Source: CAD feature listing. Evaluate the final solid. Frame: model axes, mm. A direction names the side the tool comes from. Give positions to 0.01 mm unless a question says otherwise; leave off trailing zeros. Write each loop counter-clockwise with the first axis right and the second up, starting at its lowest first coordinate (ties: lowest second). Pieces come first, ordered by that corner, then holes.
```python
from build123d import *

# Parameters (mm, degrees)
ESQUISSE1_W              = 35.4
ESQUISSE1_H              = 35.4
BOSS_EXTRU_1_DEPTH       = 14
ESQUISSE2_W              = 27.4
ESQUISSE2_H              = 27.4
ENL_V_MAT_EXTRU_1_DEPTH  = 12
ESQUISSE4_R              = 3.25
ESQUISSE4_R_2            = 1.9
BOSS_EXTRU_2_DEPTH       = 4.8
ESQUISSE5_R              = 1.75
ENL_V_MAT_EXTRU_2_DEPTH  = 2
CONG_6_R                 = 2
ESQUISSE9_W              = 1.5
ESQUISSE9_H              = 5.2
ENL_V_MAT_EXTRU_9_DEPTH  = 4
ESQUISSE8_W              = 1.5
ESQUISSE8_H              = 5.2
ENL_V_MAT_EXTRU_10_DEPTH = 4
ESQUISSE7_W              = 1.5
ESQUISSE7_H              = 5.2
ENL_V_MAT_EXTRU_11_DEPTH = 4
ESQUISSE6_W              = 1.5
ESQUISSE6_H              = 5.2
ENL_V_MAT_EXTRU_12_DEPTH = 4
ESQUISSE10_W             = 8.819289119
ESQUISSE10_H             = 5.2
ENL_V_MAT_EXTRU_13_DEPTH = 6


with BuildPart() as part:
    # Esquisse1 → Boss.-Extru.1 (new body)
    with BuildSketch(Plane(origin=(0, 0, 0), x_dir=(1, 0, 0), z_dir=(0, 1, 0))):
        Rectangle(ESQUISSE1_W, ESQUISSE1_H)
    extrude(amount=BOSS_EXTRU_1_DEPTH)

    # Esquisse2 → Enlèv. mat.-Extru.1 (cut)
    with BuildSketch(Plane(origin=(0, 14, 0), x_dir=(1, 0, 0), z_dir=(0, 1, 0))):
        Rectangle(ESQUISSE2_W, ESQUISSE2_H)
    extrude(amount=-ENL_V_MAT_EXTRU_1_DEPTH, mode=Mode.SUBTRACT)

    # Esquisse4 → Boss.-Extru.2 (add)
    # profile 1 of 4: a face of its own
    with BuildSketch(Plane(origin=(0, 2, 0), x_dir=(1, 0, 0), z_dir=(0, 1, 0))):
        with Locations(Location((-10.16, 10.16, 0), (0, 0, 270))):
            Circle(ESQUISSE4_R)
        with Locations(Location((-10.16, 10.16, 0), (0, 0, 270))):
            Circle(ESQUISSE4_R_2, mode=Mode.SUBTRACT)
    # profile 2 of 4: a face of its own
    with BuildSketch(Plane(origin=(0, 2, 0), x_dir=(1, 0, 0), z_dir=(0, 1, 0))):
        with Locations(Location((10.16, 10.16, 0), (0, 0, 270))):
            Circle(ESQUISSE4_R)
        with Locations(Location((10.16, 10.16, 0), (0, 0, 270))):
            Circle(ESQUISSE4_R_2, mode=Mode.SUBTRACT)
    # profile 3 of 4: a face of its own
    with BuildSketch(Plane(origin=(0, 2, 0), x_dir=(1, 0, 0), z_dir=(0, 1, 0))):
        with Locations(Location((10.16, -10.16, 0), (0, 0, 270))):
            Circle(ESQUISSE4_R)
        with Locations(Location((10.16, -10.16, 0), (0, 0, 270))):
            Circle(ESQUISSE4_R_2, mode=Mode.SUBTRACT)
    # profile 4 of 4: a face of its own
    with BuildSketch(Plane(origin=(0, 2, 0), x_dir=(1, 0, 0), z_dir=(0, 1, 0))):
        with Locations(Location((-10.16, -10.16, 0), (0, 0, 270))):
            Circle(ESQUISSE4_R)
        with Locations(Location((-10.16, -10.16, 0), (0, 0, 270))):
            Circle(ESQUISSE4_R_2, mode=Mode.SUBTRACT)
    extrude(amount=BOSS_EXTRU_2_DEPTH)

    # Esquisse5 → Enlèv. mat.-Extru.2 (cut)
    with BuildSketch(Plane(origin=(0, 14, 0), x_dir=(1, 0, 0), z_dir=(0, 1, 0))):
        with Locations(Location((15.5, 15.5, 0), (0, 0, 270))):
            Circle(ESQUISSE5_R)
        with Locations(Location((-15.5, 15.5, 0), (0, 0, 270))):
            Circle(ESQUISSE5_R)
        with Locations(Location((-15.5, -15.5, 0), (0, 0, 270))):
            Circle(ESQUISSE5_R)
        with Locations(Location((15.5, -15.5, 0), (0, 0, 270))):
            Circle(ESQUISSE5_R)
    extrude(amount=-ENL_V_MAT_EXTRU_2_DEPTH, mode=Mode.SUBTRACT)

    # Congé6
    cong_6_edges = [part.edges().sort_by_distance(p)[0] for p in [
        (0, 0, 17.7),
        (-17.7, 0, 0),
        (0, 0, -17.7),
        (17.7, 0, 0),
        (17.7, 7, 17.7),
        (-17.7, 7, 17.7),
        (-17.7, 7, -17.7),
        (17.7, 7, -17.7),
    ]]
    fillet(cong_6_edges, radius=CONG_6_R)

    # Esquisse9 → Enlèv. mat.-Extru.9 (cut)
    with BuildSketch(Plane(origin=(0, 0, -17.7), x_dir=(-1, 0, 0), z_dir=(0, 0, -1))):
        with Locations((-10.95, 9.4)):
            Rectangle(ESQUISSE9_W, ESQUISSE9_H)
        with Locations((-7.3, 9.4)):
            Rectangle(ESQUISSE9_W, ESQUISSE9_H)
        with Locations((-3.65, 9.4)):
            Rectangle(ESQUISSE9_W, ESQUISSE9_H)
        with Locations((0, 9.4)):
            Rectangle(ESQUISSE9_W, ESQUISSE9_H)
        with Locations((3.65, 9.4)):
            Rectangle(ESQUISSE9_W, ESQUISSE9_H)
        with Locations((7.3, 9.4)):
            Rectangle(ESQUISSE9_W, ESQUISSE9_H)
        with Locations((10.95, 9.4)):
            Rectangle(ESQUISSE9_W, ESQUISSE9_H)
    extrude(amount=-ENL_V_MAT_EXTRU_9_DEPTH, mode=Mode.SUBTRACT)

    # Esquisse8 → Enlèv. mat.-Extru.10 (cut)
    with BuildSketch(Plane.XY.offset(17.7)):
        with Locations((-10.95, 9.4)):
            Rectangle(ESQUISSE8_W, ESQUISSE8_H)
        with Locations((-7.3, 9.4)):
            Rectangle(ESQUISSE8_W, ESQUISSE8_H)
        with Locations((-3.65, 9.4)):
            Rectangle(ESQUISSE8_W, ESQUISSE8_H)
        with Locations((0, 9.4)):
            Rectangle(ESQUISSE8_W, ESQUISSE8_H)
        with Locations((3.65, 9.4)):
            Rectangle(ESQUISSE8_W, ESQUISSE8_H)
        with Locations((7.3, 9.4)):
            Rectangle(ESQUISSE8_W, ESQUISSE8_H)
        with Locations((10.95, 9.4)):
            Rectangle(ESQUISSE8_W, ESQUISSE8_H)
    extrude(amount=-ENL_V_MAT_EXTRU_10_DEPTH, mode=Mode.SUBTRACT)

    # Esquisse7 → Enlèv. mat.-Extru.11 (cut)
    with BuildSketch(Plane.ZY.offset(17.7)):
        with Locations((-10.95, 9.4)):
            Rectangle(ESQUISSE7_W, ESQUISSE7_H)
        with Locations((-7.3, 9.4)):
            Rectangle(ESQUISSE7_W, ESQUISSE7_H)
        with Locations((-3.65, 9.4)):
            Rectangle(ESQUISSE7_W, ESQUISSE7_H)
        with Locations((0, 9.4)):
            Rectangle(ESQUISSE7_W, ESQUISSE7_H)
        with Locations((3.65, 9.4)):
            Rectangle(ESQUISSE7_W, ESQUISSE7_H)
        with Locations((7.3, 9.4)):
            Rectangle(ESQUISSE7_W, ESQUISSE7_H)
        with Locations((10.95, 9.4)):
            Rectangle(ESQUISSE7_W, ESQUISSE7_H)
    extrude(amount=-ENL_V_MAT_EXTRU_11_DEPTH, mode=Mode.SUBTRACT)

    # Esquisse6 → Enlèv. mat.-Extru.12 (cut)
    with BuildSketch(Plane(origin=(17.7, 0, 0), x_dir=(0, 0, -1), z_dir=(1, 0, 0))):
        with Locations((-10.95, 9.4)):
            Rectangle(ESQUISSE6_W, ESQUISSE6_H)
        with Locations((-7.3, 9.4)):
            Rectangle(ESQUISSE6_W, ESQUISSE6_H)
        with Locations((-3.65, 9.4)):
            Rectangle(ESQUISSE6_W, ESQUISSE6_H)
        with Locations((0, 9.4)):
            Rectangle(ESQUISSE6_W, ESQUISSE6_H)
        with Locations((3.65, 9.4)):
            Rectangle(ESQUISSE6_W, ESQUISSE6_H)
        with Locations((7.3, 9.4)):
            Rectangle(ESQUISSE6_W, ESQUISSE6_H)
        with Locations((10.95, 9.4)):
            Rectangle(ESQUISSE6_W, ESQUISSE6_H)
    extrude(amount=-ENL_V_MAT_EXTRU_12_DEPTH, mode=Mode.SUBTRACT)

    # Esquisse10 → Enlèv. mat.-Extru.13 (cut)
    with BuildSketch(Plane(origin=(0, 0, -17.7), x_dir=(-1, 0, 0), z_dir=(0, 0, -1))):
        with Locations((0.009644559, 9.4)):
            Rectangle(ESQUISSE10_W, ESQUISSE10_H)
    extrude(amount=-ENL_V_MAT_EXTRU_13_DEPTH, mode=Mode.SUBTRACT)


solid = part.part
```
1. Cut plane B-B, the plane x = -5.5. Return the cut outline in (y, z).
2. Access query for faces 1 (the flat face through (7, 6.8, -16)), 2 (the cylindrical face through (-14, 13, -14.6)), 3 (the flat face through (-16, 9, 0.75)). Directions: +Z, -Z, +X, -X, +Y, -Y. A direction counts if a zero-diameter tool reaches every point of the face in a straight line with its end or side. Return the directions, or none.
3. Cut plane A-A, the plane z = 3.5. Return the cut outline in (x, y).
4. Line query: L1, parallel to X at y = 5.85, z = -10.16; L2, parallel to X at y = 12.85, z = 15.5; L3, parallel to X at y = 8.5, z = -10. Output: solid intervals per line, ascending.
5. Contact query for flat-ended pins moving along their axis: P1, Ø5, axis at x = -9, z = 9.5, coming from the +Y side; P2, Ø1.2, axis at x = 16.5, z = -0.5, coming from the -Y side; P3, Ø10, axis at x = 2, z = 6.5, coming from the +Y side. Output: stop coordinate, or through.
6. Cut plane C-C, the plane y = 9. State how many separate pieces and enclosed holes the cut face has, then the cut area to 3 significant figures.
7. Mould query, pull axis X, two halves, no side actions, for faces 4 (the cylindrical face through (11.14, 4.37, 13.26)), 5 (the flat face through (16, 12, -4)). Classes: +X half, -X half, draft (parallel to the pull), parting line (faces both ways), or undercut.
Response values:
1. outline: (0, -15.7) arc R2 ccw to (2, -17.7) - (14, -17.7) - (14, -13.7) - (2, -13.7) - (2, 13.7) - (14, 13.7) - (14, 17.7) - (2, 17.7) arc R2 ccw to (0, 15.7) - close
2. face 1: +Z, -Z
2. face 2: +Y
2. face 3: +X, -X
3. outline: (-17.7, 2) arc R2 ccw to (-15.7, 0) - (15.7, 0) arc R2 ccw to (17.7, 2) - (17.7, 6.8) - (13.7, 6.8) - (13.7, 2) - (-13.7, 2) - (-13.7, 6.8) - (-17.7, 6.8) - close; (-17.7, 12) - (-13.7, 12) - (-13.7, 14) - (-17.7, 14) - close; (13.7, 12) - (17.7, 12) - (17.7, 14) - (13.7, 14) - close
4. L1: x = -17.7 to -13.7, -13.41 to -12.06, -8.26 to -6.91, 6.91 to 8.26, 12.06 to 13.41, 13.7 to 17.7
4. L2: x = -17.7 to -17.25, -13.75 to 13.75, 17.25 to 17.7
4. L3: x = -17.7 to -13.7, 13.7 to 17.7
5. P1: stops at y = 6.8
5. P2: stops at y = 0.01
5. P3: stops at y = 2
6. separate pieces: 26
6. enclosed holes: 0
6. area: 314 mm2
7. face 4: undercut
7. face 5: draft
